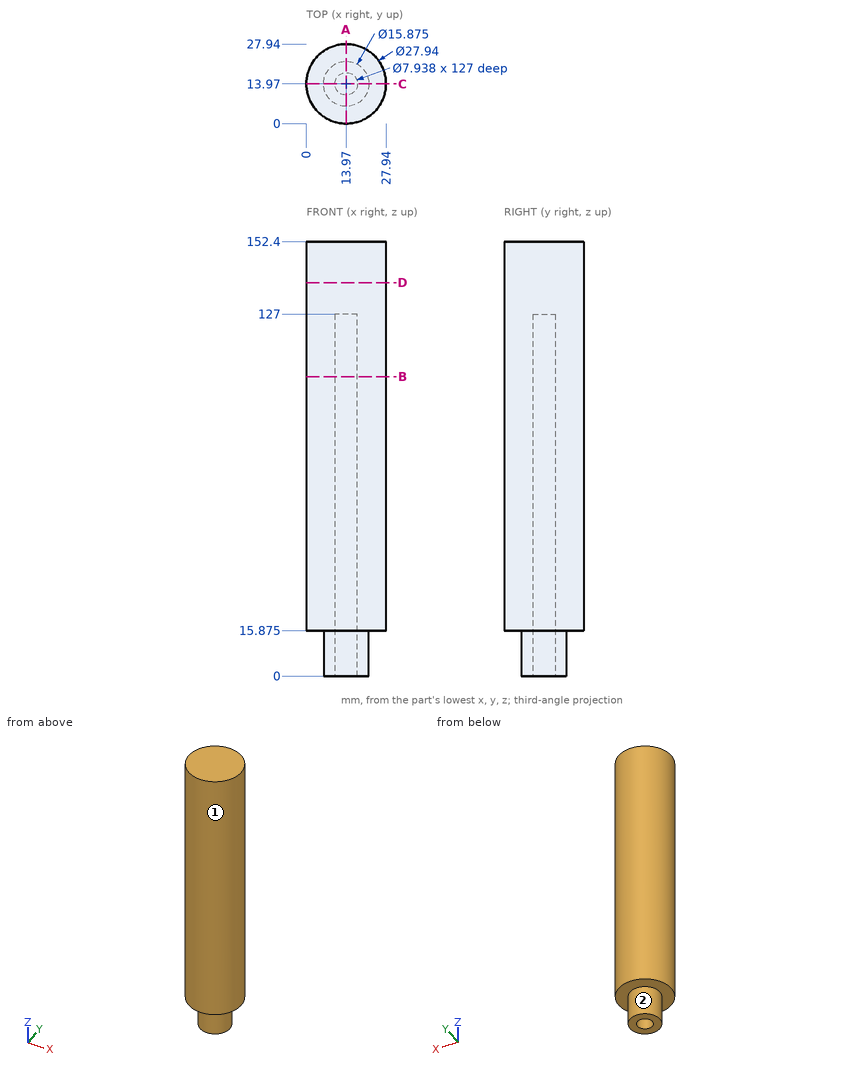
Design review of the part shown in the three views and the two pictorial views. Dimensions are in mm from the part's minimum x, y and z. A direction names the side the tool comes from. Coordinates: 2 decimals unless noted, no trailing zeros. Order: outer loops, then holes, each group sorted by start corner. A loop starts at its lowest first (then second) coordinate and runs counter-clockwise, first axis right, second up. Notation, with made-up numbers: (38.5, 54.25) - (94.5, 54.25) arc R24 ccw to (94.5, 64.25) - close; hole circle Ø4 at (37, 32.25). An arc over 180 degrees is marked (long way). Answer as CSV lines item,"result". Start each with the question number.
1) Add section B-B (z = 105). State the section outline as (x, y) points, then the cut area to 3 significant figures.
2) Machinability: for the marked faces 1 and 2, which of the approach directions +Z, -Z, +X, -X, +Y, -Y give a long, thin tool a straight path to every point of the face, cutting with its end or side? Answer none if there is none.
3) Add section D-D (z = 138). State the section outline as (x, y) points.
4) Add section A-A (x = 13.97). State the section outline as (y, z) points (1 decimal).
5) To check wall thickness, follow line 1 along Y through (x, z) = (13.97, 72.5); line 2 along Z through (x, y) = (19, 26.75) (1 decimal). State the ranges of each line that lie inside material, in increasing order. Write a range as [from, to].
6) Insertion check: P1, Ø3, axis at y = 5.5, z = 132, coming from the +X side; P2, Ø14, axis at x = 7.5, y = 8.5, coming from the -Z side; P3, Ø8, axis at y = 9.5, z = 60, coming from the -X side; P4, Ø3, axis at x = 3.5, z = 97, coming from the +Y side. Each pin has a flat end and moves straight along its axis. Give the tip position at first contact, or say it passes through.
Result:
1,outline,"circle Ø27.94 at (13.97, 13.97); hole circle Ø7.94 at (13.97, 13.97)"
1,area,"564 mm^2"
2,face 1,"+Z, -Z"
2,face 2,"-Z"
3,outline,"circle Ø27.94 at (13.97, 13.97)"
4,outline,"(0, 15.9) - (6, 15.9) - (6, 0) - (10, 0) - (10, 127) - (17.9, 127) - (17.9, 0) - (21.9, 0) - (21.9, 15.9) - (27.9, 15.9) - (27.9, 152.4) - (0, 152.4) - close"
5,line 1,"[0, 10], [17.94, 27.94]"
5,line 2,"[15.9, 152.4]"
6,P1,"x = 26.08"
6,P2,"z = 0"
6,P3,"x = 0.01"
6,P4,"y = 24.68"
